The listing builds one solid part. Answer for the finished solid, in the listing's coordinates (mm). Face numbers are marked on the shaded views. A direction names the side the tool comes from. Give positions to 0.01 mm unless a question says otherwise; leave off trailing zeros. Order: outer loops, then holes, each group sorted by start corner. A loop starts at its lowest first (then second) coordinate and runs counter-clockwise, first axis right, second up. Notation, with made-up numbers: (59, 1) - (88, 1) arc R31 cw to (88, 29) - close; hole circle Ø4 at (62, 52). An arc over 180 degrees is marked (long way). Answer as a JSON object with one key per item and string values. Group by question number.
Q1. A cutting plane is placed at D-D, the plane z = -3.25. Give the vertices of the cut face in (x, y) (3 decimals).
Q2. The mould has two halves that part along Y. Classify the marked faces 1, 2 and 3: released by +Y, released by -Y, zero draft, split by the parting line, or undercut.
Q3. For the marked faces 4 and 5, determine the directions among +Z, -Z, +X, -X, +Y, -Y from which every point of the face is accessible in a straight line to the end or side of a thin tool.
Q4. Given pin 1 (5 mm diameter, centred on x = 6.45, z = 0, fed in from +Y); pin 2 (3 mm diameter, centred on x = -12.9, y = 3.275, fed in from -Z) (3 decimals); pin 3 (4 mm diameter, centred on x = 12, z = -2.5, fed in from +Y), each flat-ended and moving along its own axis, determine where each tip first touches the part or whether it passes through.
Q5. Consider line 1 (X direction, y = 2.5, z = 0); line 2 (X direction, y = 4, z = -3.75); line 3 (Y direction, x = 0, z = -3.75) (3 decimals). Determine where each line is inside the solid, lowest interval first.
Q6. A cutting plane is placed at B-B, the plane x = 0. Give the vertices of the cut face in (y, z) (3 decimals).
Q7. A cutting plane is placed at A-A, the plane z = 0. Give the vertices of the cut face in (x, y).
Q8. A cutting plane is placed at C-C, the plane x = 10.5. Give the vertices of the cut face in (y, z), and give its area (3 significant figures).
from build123d import *

# Parameters (mm, degrees)
SKETCH1_W           = 33.3
SKETCH1_H           = 8.9
SKETCH1_R           = 2.7
BOSS_EXTRUDE1_DEPTH = 6.55
CUT_EXTRUDE1_REACH  = 10.9
SKETCH2_R           = 2


with BuildPart() as part:
    # Sketch1 → Boss-Extrude1 (new body)
    with BuildSketch(Plane(origin=(0, 0, 0), x_dir=(1, 0, 0), z_dir=(0, 1, 0))):
        Rectangle(SKETCH1_W, SKETCH1_H)
        with Locations((-12.9, 0)):
            Circle(SKETCH1_R, mode=Mode.SUBTRACT)
        with Locations((-6.45, 0)):
            Circle(SKETCH1_R, mode=Mode.SUBTRACT)
        Circle(SKETCH1_R, mode=Mode.SUBTRACT)
        with Locations((6.45, 0)):
            Circle(SKETCH1_R, mode=Mode.SUBTRACT)
        with Locations((12.9, 0)):
            Circle(SKETCH1_R, mode=Mode.SUBTRACT)
    extrude(amount=BOSS_EXTRUDE1_DEPTH)

    # Sketch2 → Cut-Extrude1 (cut, up to next)
    with BuildSketch(Plane(origin=(0, 0, -4.45), x_dir=(-1, 0, 0), z_dir=(0, 0, -1)), mode=Mode.PRIVATE) as cut_extrude1_sk1:
        with Locations((-12.9, 3.275)):
            Circle(SKETCH2_R)
    cut_extrude1_tool1 = extrude(cut_extrude1_sk1.sketch, amount=-CUT_EXTRUDE1_REACH, mode=Mode.PRIVATE) & part.part
    add(cut_extrude1_tool1.solids().sort_by_distance((12.9, 3.275, -4.45))[0], mode=Mode.SUBTRACT)
    # Sketch2 → Cut-Extrude1 (cut, up to next)
    with BuildSketch(Plane(origin=(0, 0, -4.45), x_dir=(-1, 0, 0), z_dir=(0, 0, -1)), mode=Mode.PRIVATE) as cut_extrude1_sk2:
        with Locations((-6.45, 3.275)):
            Circle(SKETCH2_R)
    cut_extrude1_tool2 = extrude(cut_extrude1_sk2.sketch, amount=-CUT_EXTRUDE1_REACH, mode=Mode.PRIVATE) & part.part
    add(cut_extrude1_tool2.solids().sort_by_distance((6.45, 3.275, -4.45))[0], mode=Mode.SUBTRACT)
    # Sketch2 → Cut-Extrude1 (cut, up to next)
    with BuildSketch(Plane(origin=(0, 0, -4.45), x_dir=(-1, 0, 0), z_dir=(0, 0, -1)), mode=Mode.PRIVATE) as cut_extrude1_sk3:
        with Locations((0, 3.275)):
            Circle(SKETCH2_R)
    cut_extrude1_tool3 = extrude(cut_extrude1_sk3.sketch, amount=-CUT_EXTRUDE1_REACH, mode=Mode.PRIVATE) & part.part
    add(cut_extrude1_tool3.solids().sort_by_distance((0, 3.275, -4.45))[0], mode=Mode.SUBTRACT)
    # Sketch2 → Cut-Extrude1 (cut, up to next)
    with BuildSketch(Plane(origin=(0, 0, -4.45), x_dir=(-1, 0, 0), z_dir=(0, 0, -1)), mode=Mode.PRIVATE) as cut_extrude1_sk4:
        with Locations((6.45, 3.275)):
            Circle(SKETCH2_R)
    cut_extrude1_tool4 = extrude(cut_extrude1_sk4.sketch, amount=-CUT_EXTRUDE1_REACH, mode=Mode.PRIVATE) & part.part
    add(cut_extrude1_tool4.solids().sort_by_distance((-6.45, 3.275, -4.45))[0], mode=Mode.SUBTRACT)
    # Sketch2 → Cut-Extrude1 (cut, up to next)
    with BuildSketch(Plane(origin=(0, 0, -4.45), x_dir=(-1, 0, 0), z_dir=(0, 0, -1)), mode=Mode.PRIVATE) as cut_extrude1_sk5:
        with Locations((12.9, 3.275)):
            Circle(SKETCH2_R)
    cut_extrude1_tool5 = extrude(cut_extrude1_sk5.sketch, amount=-CUT_EXTRUDE1_REACH, mode=Mode.PRIVATE) & part.part
    add(cut_extrude1_tool5.solids().sort_by_distance((-12.9, 3.275, -4.45))[0], mode=Mode.SUBTRACT)


solid = part.part
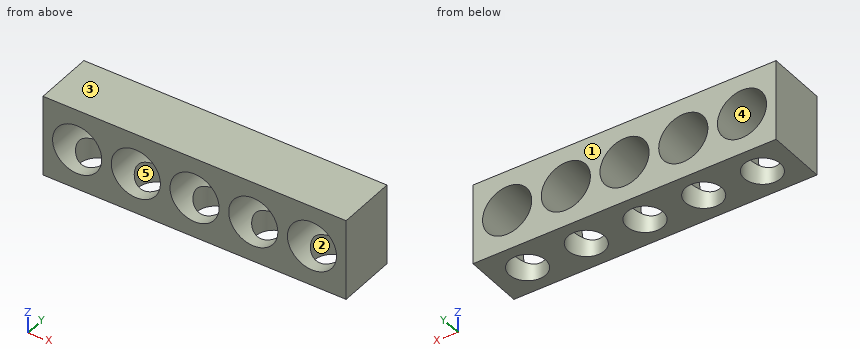
Reply:
{
 "1": {"outline": "(-16.65, 0) - (16.65, 0) - (16.65, 6.55) - (-16.65, 6.55) - close; hole circle Ø4 at (-12.9, 3.275); hole circle Ø4 at (-6.45, 3.275); hole circle Ø4 at (0, 3.275); hole circle Ø4 at (6.45, 3.275); hole circle Ø4 at (12.9, 3.275)"},
 "2": {"face 1": "released by +Y", "face 2": "undercut", "face 3": "zero draft"},
 "3": {"face 4": "+Y, -Y", "face 5": "-Z"},
 "4": {"pin 1": "passes through", "pin 2": "stops at z = 2.245", "pin 3": "stops at y = 6.55"},
 "5": {"line 1": "x = -16.65 to -15.6, -10.2 to -9.15, -3.75 to -2.7, 2.7 to 3.75, 9.15 to 10.2, 15.6 to 16.65", "line 2": "x = -16.65 to -14.76, -11.04 to -8.31, -4.59 to -1.86, 1.86 to 4.59, 8.31 to 11.04, 14.76 to 16.65", "line 3": "y = 0 to 1.275, 5.275 to 6.55"},
 "6": {"outline": "(0, -4.45) - (1.275, -4.45) - (1.275, -2.7) - (0, -2.7) - close; (0, 2.7) - (6.55, 2.7) - (6.55, 4.45) - (0, 4.45) - close; (5.275, -4.45) - (6.55, -4.45) - (6.55, -2.7) - (5.275, -2.7) - close"},
 "7": {"outline": "(-16.65, 0) - (-15.6, 0) - (-15.6, 6.55) - (-16.65, 6.55) - close; (-10.2, 0) - (-9.15, 0) - (-9.15, 6.55) - (-10.2, 6.55) - close; (-3.75, 0) - (-2.7, 0) - (-2.7, 6.55) - (-3.75, 6.55) - close; (2.7, 0) - (3.75, 0) - (3.75, 6.55) - (2.7, 6.55) - close; (9.15, 0) - (10.2, 0) - (10.2, 6.55) - (9.15, 6.55) - close; (15.6, 0) - (16.65, 0) - (16.65, 6.55) - (15.6, 6.55) - close"},
 "8": {"outline": "(0, -4.45) - (6.55, -4.45) - (6.55, -1.24) - (0, -1.24) - close; (0, 1.24) - (6.55, 1.24) - (6.55, 4.45) - (0, 4.45) - close", "area": "42.1 mm^2"}
}
